Study the drawing (mm; zero at the part's minimum x, y, z) and answer. A direction names the side the tool comes from. Coordinates: 2 decimals unless noted, no trailing zeros. Loops run counter-clockwise (first coordinate to the right, second up) from the corner with the lowest first, then second, coordinate; pieces in that order, holes last. Notation, with made-up numbers: (30.5, -37.5) -> (85.5, -37.5) arc R32 ccw to (85.5, -9.5) -> close; hole circle Ø8 at (9.5, -16.75). An arc over 180 degrees is marked (long way). Answer in a Markdown table with one row per item.
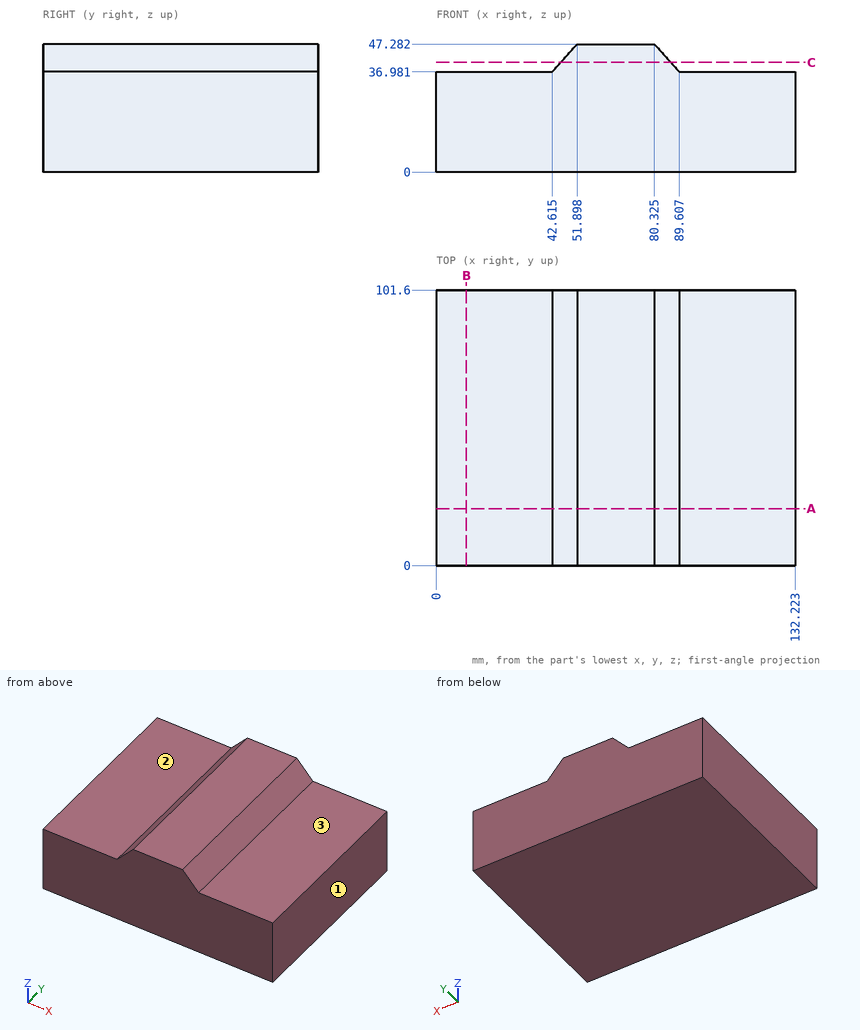
1. Given pin 1 Ø13 at (x, y) = (118.5, 39) entering from +Z, flat-ended and moving along its own axis, determine where the tip first touches the part or whether it passes through.
A:
| item | result |
|---|---|
| pin 1 | stops at z = 36.98 |
2. A cutting plane is placed at C-C on z = 40.5. Give the vertices of the cut face in (x, y), and give its area (3 significant figures).
A:
| item | result |
|---|---|
| outline | (45.79, 0) -> (86.44, 0) -> (86.44, 101.6) -> (45.79, 101.6) -> close |
| area | 4,130 mm2 |
3. A cutting plane is placed at A-A on y = 21. Give the vertices of the cut face in (x, z) (1 decimal).
A:
| item | result |
|---|---|
| outline | (0, 0) -> (132.2, 0) -> (132.2, 37) -> (89.6, 37) -> (80.3, 47.3) -> (51.9, 47.3) -> (42.6, 37) -> (0, 37) -> close |
4. Find the intervals of material crossed by probe 1 along Z at (x, y) = (126, 52); probe 2 along Z at (x, y) = (89.5, 83.5); probe 3 along X at (y, z) = (29.5, 39) (1 decimal), in increasing order.
A:
| item | result |
|---|---|
| probe 1 | z = 0 to 36.98 |
| probe 2 | z = 0 to 37.1 |
| probe 3 | x = 44.4 to 87.8 |
5. A tool of negligible diameter and unlimited length cuts with its end or side. For the marked faces 1, 2 and 3, from which of +Z, -Z, +X, -X, +Y, -Y can it reach the whole face along a straight path? Write none if from no direction.
A:
| item | result |
|---|---|
| face 1 | +Z, -Z, +X, +Y, -Y |
| face 2 | +Z, -X, +Y, -Y |
| face 3 | +Z, +X, +Y, -Y |
6. A cutting plane is placed at B-B on x = 11. Give the vertices of the cut face in (y, z), and give its area (3 significant figures).
A:
| item | result |
|---|---|
| outline | (0, 0) -> (101.6, 0) -> (101.6, 36.98) -> (0, 36.98) -> close |
| area | 3,760 mm2 |
